CAD build for the part. Positions are in the model's coordinates, mm. Round coordinates to 2 decimals unless told otherwise and drop trailing zeros. Loops run counter-clockwise (first coordinate to the right, second up) from the corner with the lowest first, then second, coordinate; pieces in that order, holes last. Notation, with made-up numbers: (55, 3) - (112, 3) arc R29 cw to (112, 32) - close; hole circle Ø4 at (9.5, 44.5). An arc over 180 degrees is marked (long way). One line per question, with ' | ' between items.
```python
from build123d import *

# Parameters (mm, degrees)
BASPROSKE_W         = 12
BASPROSKE_H         = 6.5
TOOTHCUT_DEPTH      = 16.116216458
TEETHCUTS_COUNT     = 11
TEETHCUTS_ANGLE     = 327.272727273
BORSKE_R            = 2.5
BORE_DEPTH          = 50.0000508
BOSS_EXTRUDE1_DEPTH = 12


with BuildPart() as part:
    # BasProSke → Base-Revolve (revolve)
    with BuildSketch(Plane(origin=(0, 0, 0), x_dir=(1, 0, 0), z_dir=(0, 1, 0)), mode=Mode.PRIVATE) as base_revolve_sk:
        with Locations((6, 3.25)):
            Rectangle(BASPROSKE_W, BASPROSKE_H)
    revolve(base_revolve_sk.sketch.rotate(Axis((-10, 0, 0), (1, 0, 0)), 180), axis=Axis((-10, 0, 0), (1, 0, 0)))

    # TooCutSke → ToothCut (cut, through all)
    with BuildSketch(Plane(origin=(0, 0, 0), x_dir=(0, 0, -1), z_dir=(1, 0, 0))):
        with BuildLine():
            ThreePointArc((0.576045815, 4.209771041), (0, 4.249), (-0.576045815, 4.209771041))
            ThreePointArc((-0.576045815, 4.209771041), (-0.841371334, 5.420048739), (-1.718652745, 6.295004202))
            ThreePointArc((-1.718652745, 6.295004202), (0, 6.5254), (1.718652745, 6.295004202))
            ThreePointArc((1.718652745, 6.295004202), (0.841371334, 5.420048739), (0.576045815, 4.209771041))
        make_face()
    toothcut = extrude(amount=TOOTHCUT_DEPTH, mode=Mode.SUBTRACT)

    # TeethCuts: ToothCut ×11 about axis
    teethcuts_axis = Axis((-10, 0, 0), (1, 0, 0))
    for i in range(1, TEETHCUTS_COUNT):
        add(toothcut.rotate(teethcuts_axis, i * TEETHCUTS_ANGLE / (TEETHCUTS_COUNT - 1)), mode=Mode.SUBTRACT)

    # BorSke → Bore (cut, symmetric)
    with BuildSketch(Plane(origin=(0, 0, 0), x_dir=(0, 0, -1), z_dir=(1, 0, 0))):
        with Locations(Location((0, 0, 0), (0, 0, 180))):
            Circle(BORSKE_R)
    extrude(amount=BORE_DEPTH, both=True, mode=Mode.SUBTRACT)

    # Sketch1 → Boss-Extrude1 (add)
    with BuildSketch(Plane(origin=(12, 0, 0), x_dir=(0, 0, -1), z_dir=(1, 0, 0))):
        with BuildLine():
            Line((-1.1, 2.244994432), (1.1, 2.244994432))
            ThreePointArc((1.1, 2.244994432), (0, 2.5), (-1.1, 2.244994432))
        make_face()
    extrude(amount=-BOSS_EXTRUDE1_DEPTH)


solid = part.part
```
(1) Cut at A-A, the plane z = 4.5. Write the cut outline in (x, y), then the cut area to 3 significant figures.
Results found:
outline: (0, -2.88) - (12, -2.88) - (12, -1.24) - (0, -1.24) - close; (0, -0.07) - (12, -0.07) - (12, 1.4) - (0, 1.4) - close; (0, 2.92) - (12, 2.92) - (12, 4.36) - (0, 4.36) - close | area: 54.7 mm²
(2) Two-plate mould, pull along X, no slides. Class faces 1 (the face through (0, 3, 0)), 2 (the face through (6.1, -2.5, 0.1)): released by +X, released by -X, zero draft, split by the parting line, or undercut.
Results found:
face 1: released by -X | face 2: zero draft
(3) Cut at B-B, the plane y = -0.75. Write the cut outline in (x, z).
Results found:
outline: (0, -4.18) - (12, -4.18) - (12, -2.38) - (0, -2.38) - close; (0, 2.38) - (12, 2.38) - (12, 4.18) - (0, 4.18) - close
(4) Drop flat-ended pins along their axis: P1, Ø4, axis at x = 4.5, y = 3, coming from the +Z side; P2, Ø3, axis at x = 5, y = -4, coming from the -Z side; P3, Ø3, axis at x = 1.5, y = 4.5, coming from the +Z side. Give the stop position or say it passes through.
Results found:
P1: stops at z = 6.42 | P2: stops at z = -5.97 | P3: stops at z = 5.01
(5) Cut at C-C, the plane y = -4.75. Write the cut outline in (x, z).
Results found:
outline: (0, -3.67) - (12, -3.67) - (12, -2.15) - (0, -2.15) - close; (0, -0.76) - (12, -0.76) - (12, 0.76) - (0, 0.76) - close; (0, 2.15) - (12, 2.15) - (12, 3.67) - (0, 3.67) - close
(6) Probe L1, parallel to Z at x = 4.75, y = -5; L2, parallel to Z at x = 8, y = -2.75; L3, parallel to Z at x = 8.5, y = 0.75. List the from-to ranges inside material, lowest first.
Results found:
L1: z = -3.68 to -2.37, -0.77 to 0.77, 2.37 to 3.68 | L2: z = -5.89 to -4.17, -3.24 to 3.24, 4.17 to 5.89 | L3: z = -6.43 to -2.38, 2.38 to 6.43
